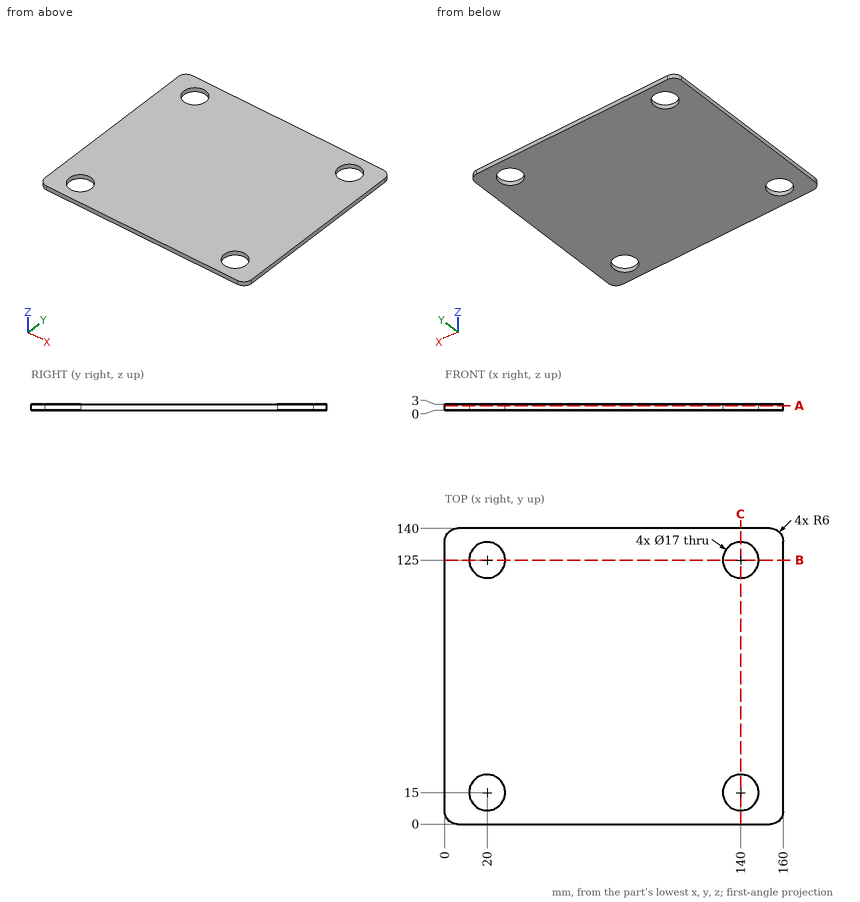
Check sheet for the drawn part. Datum: minimum x, y, z corner. Units: mm. Give positions to 0.01 mm unless a question says otherwise; leave off trailing zeros. Write each loop counter-clockwise with the first axis right and the second up, starting at its lowest first coordinate (ties: lowest second). Pieces come first, ordered by that corner, then holes. Notation, with made-up numbers: (84, 56.5) -> (137, 56.5) arc R25 ccw to (137, 92.5) -> close; hole circle Ø10 at (22, 42.25). An arc over 180 degrees is marked (long way). Use one line per item in the form item = value. Start each with the question number.
1. Section check C-C (x = 140). Record the cut outline in (y, z), and give its area (3 significant figures).
2. Section check A-A (z = 2.2). Record the cut outline in (x, y), and give its area (3 significant figures).
3. Go/stop test with flat-tipped pins: P1, Ø15.5, axis at x = 140, y = 125, coming from the -Z side; P2, Ø1.5, axis at x = 60, y = 48, coming from the -Z side. Record where each tip stops, or that it passes through.
4. Thickness scan on line 1 along Y through (x, z) = (20, 1.05); line 2 along X through (y, z) = (122, 1.7); line 3 along Y through (x, z) = (138.5, 0.4). Record the ranges inside material, lowest first. Write a range as from..to.
5. Section check B-B (y = 125). Record the cut outline in (x, z), and give its area (3 significant figures).
Conclusion:
q1.outline = (0, 0) -> (6.5, 0) -> (6.5, 3) -> (0, 3) -> close; (23.5, 0) -> (116.5, 0) -> (116.5, 3) -> (23.5, 3) -> close; (133.5, 0) -> (140, 0) -> (140, 3) -> (133.5, 3) -> close
q1.area = 318 mm²
q2.outline = (0, 6) arc R6 ccw to (6, 0) -> (154, 0) arc R6 ccw to (160, 6) -> (160, 134) arc R6 ccw to (154, 140) -> (6, 140) arc R6 ccw to (0, 134) -> close; hole circle Ø17 at (20, 15); hole circle Ø17 at (20, 125); hole circle Ø17 at (140, 15); hole circle Ø17 at (140, 125)
q2.area = 21,500 mm²
q3.P1 = through
q3.P2 = 0
q4.line_1 = 0..6.5, 23.5..116.5, 133.5..140
q4.line_2 = 0..12.05, 27.95..132.05, 147.95..160
q4.line_3 = 0..6.63, 23.37..116.63, 133.37..140
q5.outline = (0, 0) -> (11.5, 0) -> (11.5, 3) -> (0, 3) -> close; (28.5, 0) -> (131.5, 0) -> (131.5, 3) -> (28.5, 3) -> close; (148.5, 0) -> (160, 0) -> (160, 3) -> (148.5, 3) -> close
q5.area = 378 mm²
